For this review, take the finished solid that the model builds, in its own axes (mm). Round coordinates to 2 decimals unless told otherwise and drop trailing zeros. Order: outer loops, then holes, each group sorted by start corner. A loop starts at its lowest first (then second) coordinate and runs counter-clockwise, first axis right, second up. Notation, with made-up numbers: M 14,-39 L 63,-39 A21 cw 63,-4 Z; hole C -26,-36 d2. An arc over 180 degrees is marked long. Use a Markdown table: item, result.
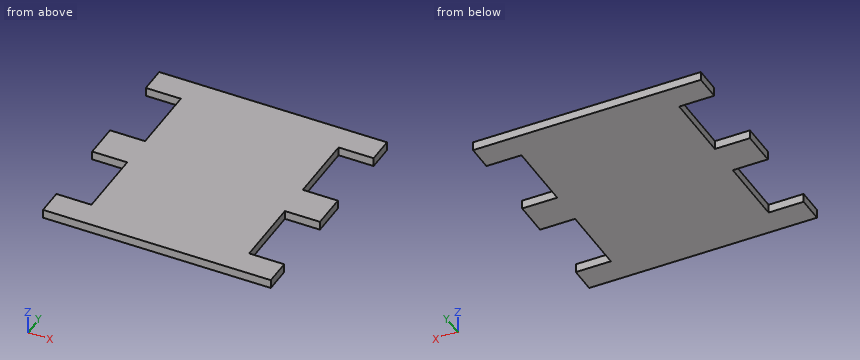
from build123d import *

# Parameters (mm, degrees)
ESQUISSE1_W             = 130
ESQUISSE1_H             = 130
BOSS_EXTRU_1_DEPTH      = 5
ESQUISSE2_W             = 20
ESQUISSE2_H             = 40
ENL_V_MAT_EXTRU_1_DEPTH = 10
ESQUISSE3_W             = 20
ESQUISSE3_H             = 40
ENL_V_MAT_EXTRU_2_DEPTH = 10


with BuildPart() as part:
    # Esquisse1 → Boss.-Extru.1 (new body)
    with BuildSketch(Plane.XY):
        with Locations((31.574099396, -23.428129952)):
            Rectangle(ESQUISSE1_W, ESQUISSE1_H)
    extrude(amount=BOSS_EXTRU_1_DEPTH)

    # Esquisse2 → Enlèv. mat.-Extru.1 (cut)
    with BuildSketch(Plane.XY.offset(5)):
        with Locations((-23.425900604, 6.571870048)):
            Rectangle(ESQUISSE2_W, ESQUISSE2_H)
        with Locations((-23.425900604, -53.428129952)):
            Rectangle(ESQUISSE2_W, ESQUISSE2_H)
    extrude(amount=-ENL_V_MAT_EXTRU_1_DEPTH, mode=Mode.SUBTRACT)

    # Esquisse3 → Enlèv. mat.-Extru.2 (cut)
    with BuildSketch(Plane.XY.offset(5)):
        with Locations((86.574099396, 6.571870048)):
            Rectangle(ESQUISSE3_W, ESQUISSE3_H)
        with Locations((86.574099396, -53.428129952)):
            Rectangle(ESQUISSE3_W, ESQUISSE3_H)
    extrude(amount=-ENL_V_MAT_EXTRU_2_DEPTH, mode=Mode.SUBTRACT)


solid = part.part
Q1. Add section A-A (z = 3.2). Write out the cut boundary in (x, y), then the cut area to 3 significant figures.
Determined:
| item | result |
|---|---|
| outline | M -33.43,-88.43 L 96.57,-88.43 L 96.57,-73.43 L 76.57,-73.43 L 76.57,-33.43 L 96.57,-33.43 L 96.57,-13.43 L 76.57,-13.43 L 76.57,26.57 L 96.57,26.57 L 96.57,41.57 L -33.43,41.57 L -33.43,26.57 L -13.43,26.57 L -13.43,-13.43 L -33.43,-13.43 L -33.43,-33.43 L -13.43,-33.43 L -13.43,-73.43 L -33.43,-73.43 Z |
| area | 13,700 mm^2 |
Q2. Wall thickness on line 1 along Y through (x, z) = (81, 1.4); line 2 along X through (y, z) = (-50.5, 3.75): over which ranges is each line inside the solid? List them lowest first. Write a range as [from, to].
Determined:
| item | result |
|---|---|
| line 1 | y = [-88.43, -73.43], [-33.43, -13.43], [26.57, 41.57] |
| line 2 | x = [-13.43, 76.57] |
Q3. Add section B-B (y = -43.5). Write out the cut boundary in (x, z).
Determined:
| item | result |
|---|---|
| outline | M -13.43,0 L 76.57,0 L 76.57,5 L -13.43,5 Z |
